Autodesk Inventor part; units mm, degrees
ref_plane "Work Plane1" through (-47.8192, -31.25, -6) normal (0, 0, 1) x (1, 0, 0)
ref_plane "YZ Plane" through (0, 0, 0) normal (1, 0, 0) x (0, 1, 0)
ref_plane "XZ Plane" through (0, 0, 0) normal (0, 1, 0) x (-1, 0, 0)
sketch "Sketch1" plane through (0, 0, 0) normal (0, 0, 1) x (1, 0, 0)
  circle A0 centre (-53.184, -21.25) radius 1.5
  arc A1 (-60.184, 31.25) -> (-62.184, 29.25) centre (-60.184, 29.25) ccw
  line L0 (-62.184, -29.25) -> (-62.184, 29.25)
  arc A2 (-62.184, -29.25) -> (-60.184, -31.25) centre (-60.184, -29.25) ccw
  line L1 (-47.8192, -31.25) -> (-60.184, -31.25)
  line L2 (-47.8192, -31.25) -> (-47.8192, 31.25)
  line L3 (-47.8192, 31.25) -> (-60.184, 31.25)
  circle A3 centre (-53.184, 21.25) radius 1.5
  circle A4 centre (27.484, 0) radius 1.5
  circle A5 centre (-53.184, 21.25) radius 2
  circle A6 centre (-53.184, 21.25) radius 1
  circle A7 centre (-53.184, -21.25) radius 1
  circle A8 centre (-53.184, -21.25) radius 2
  circle A9 centre (27.484, 0) radius 2
  circle A10 centre (27.484, 0) radius 1
  line L4 (-52.6745, 23.184) -> (27.9935, 1.934)
  line L5 (27.9935, -1.934) -> (-52.6745, -23.184)
  line L6 (-55.184, -21.25) -> (-55.184, 21.25)
  arc A11 (-52.6745, 23.184) -> (-55.184, 21.25) centre (-53.184, 21.25) ccw
  arc A12 (-55.184, -21.25) -> (-52.6745, -23.184) centre (-53.184, -21.25) ccw
  arc A13 (27.9935, -1.934) -> (27.9935, 1.934) centre (27.484, 0) ccw
  point P0 (0, 0)
  dimension "d0" = 4
  dimension "d1" = 4
  dimension "d2" = 4
  dimension "d3" = 2
extrude "Extrusion1" add sketch "Sketch1" along normal blind 9 contours A0 | A5 | A9 | A8 | A3 | A4
extrude "Extrusion2" add sketch "Sketch1" along normal blind 4 contours L4 A9 L5 L2 | L2 L5 A8 L6 A5 L4
sketch "Sketch2" plane through (0, 0, 0) normal (0, 0, -1) x (-1, 0, 0)
  line L0 (-22.1808, 31.25) -> (-22.1808, -31.25)
  line L1 (47.8192, 31.25) -> (-22.1808, 31.25)
  line L2 (47.8192, -31.25) -> (47.8192, 31.25)
  line L3 (-22.1808, -31.25) -> (47.8192, -31.25)
  line L4 (47.8192, -21.905) -> (47.8192, 21.905)
  line L5 (47.8192, 21.905) -> (-22.1808, 3.4652)
  line L6 (-22.1808, 3.4652) -> (-22.1808, -3.4652)
  line L7 (-22.1808, -3.4652) -> (47.8192, -21.905)
  line L8 (52.6745, 23.184) -> (-27.9935, 1.934)
  line L9 (-27.9935, -1.934) -> (52.6745, -23.184)
  line L10 (47.7192, -21.8787) -> (47.7192, 21.8787)
  line L11 (47.7192, 21.7753) -> (-22.0808, 3.3882)
  line L12 (-22.0808, 3.4916) -> (-22.0808, -3.4916)
  line L13 (-22.0808, -3.3882) -> (47.7192, -21.7753)
  line L14 (47.7192, 21.7753) -> (47.7192, 21.8787)
  line L15 (-22.0808, 3.3882) -> (-22.0808, 3.4916)
  line L16 (47.8192, 21.905) -> (-22.1808, 3.4652)
  point P0 (0, 0)
  point P1 (-22.1808, 0)
  dimension "d8" = 0.1
  dimension "d11" = 0.1
  dimension "d12" = 0.1
  dimension "d13" = 0.1
ref_plane "Work Plane1" through (-47.8192, -31.25, -6) normal (0, 0, 1) x (1, 0, 0)
extrude "Extrusion3" add sketch "Sketch2" along normal up to surface (6 mm away) contours L5 L10 L11 L12 | L12 L13 L10 L7 | L11 L10 L13 L12
properties part number "3d_LM-Welding_Tooling - Top Adapter" material "PA12 SLS 3D Print"
Input: part model. Units: mm. Frame: model coordinates. A direction names the side the tool comes from. Give positions to 0.01 mm unless a question says otherwise; leave off trailing zeros. Order: outer loops, then holes, each group sorted by start corner. A loop starts at its lowest first (then second) coordinate and runs counter-clockwise, first axis right, second up. Notation, with made-up numbers: (-7.5, 66) -> (34.5, 66) arc R22 ccw to (34.5, 92) -> close; hole circle Ø11 at (6.5, -18). An arc over 180 degrees is marked (long way). Use one line per item in the form item = value.
1) Section B-B, the plane y = -18. Return loops of the section in (x, z), and give its area (3 significant figures).
Response values:
outline = (-55.18, 0) -> (-47.72, 0) -> (-47.72, -6) -> (-33, -6) -> (-33, 4) -> (-55.18, 4) -> close
area = 177 mm^2
2) Mould query, pull axis Y, two halves, no side actions, for faces 1 (the flat face through (22.081, 0, -3)), 2 (the cylindrical face through (-53.978, -20.642, 4.437)), 3 (the cylindrical face through (29.39, -0.6, 5.44)). Classes: pulls with the +Y half, pulls with the -Y half, needs draft (parallel to the pull), parting line crosses it, or undercut.
Response values:
face_1 = needs draft
face_2 = undercut
face_3 = parting line crosses it
3) Section C-C, the plane x = -27. Return loops of the section in (y, z).
Response values:
outline = (-16.42, -6) -> (16.42, -6) -> (16.42, 4) -> (-16.42, 4) -> close
4) First-contact query: pin 1 Ø5 at (y, z) = (-10.5, -3.5) entering from -X; pin 2 Ø3 at (x, y) = (-36, 7.5) entering from +Z; pin 3 Ø5.5 at (x, y) = (25, 0) entering from -Z; pin 4 Ø3 at (x, y) = (27.484, 0) entering from +Z. Flat tips, straight axial feed; report the tip coordinate or a pass-through.
Response values:
pin_1 = -47.72
pin_2 = 4
pin_3 = 0
pin_4 = 9
5) Line query: probe 1 along Z at (x, y) = (-20.5, 1); probe 2 along Z at (x, y) = (-51, -6.5); probe 3 along Y at (x, z) = (-41.5, 3). Output: solid intervals per line, ascending.
Response values:
probe_1 = -6 to 4
probe_2 = 0 to 4
probe_3 = -20.24 to 20.24
6) Reachability of faces 4 (the flat face through (-52, 0, 0)), 5 (the cylindrical face through (-53.978, 21.858, 4.437)), 6 (the flat face through (28.3, -0.9, 9)), 7 (the cylindrical face through (-54.66, -22.6, 5.44)), 8 (the flat face through (25, 0, 0)) from +Z, -Z, +X, -X, +Y, -Y: full face, straight path, thin tool, end or side. Return the list, or none.
Response values:
face_4 = -Z, -X, +Y, -Y
face_5 = +Z, -Z
face_6 = +Z, +X, -X, +Y, -Y
face_7 = +Z
face_8 = -Z, +X, +Y, -Y
7) Section A-A, the plane y = 0. Return loops of the section in (x, z), and give its area (3 significant figures).
Response values:
outline = (-55.18, 0) -> (-47.72, 0) -> (-47.72, -6) -> (22.08, -6) -> (22.08, 0) -> (26.48, 0) -> (26.48, 9) -> (25.48, 9) -> (25.48, 4) -> (-55.18, 4) -> close; (28.48, 0) -> (29.48, 0) -> (29.48, 9) -> (28.48, 9) -> close
area = 759 mm^2
8) Section D-D, the plane y = 16. Return loops of the section in (x, z).
Response values:
outline = (-55.18, 0) -> (-47.72, 0) -> (-47.72, -6) -> (-25.4, -6) -> (-25.4, 4) -> (-55.18, 4) -> close
